Geometry: final body of the model. Coordinates: model frame, mm. A direction names the side the tool comes from. Round coordinates to 2 decimals unless told otherwise and drop trailing zeros. Write each loop counter-clockwise with the first axis right and the second up, starting at its lowest first coordinate (ties: lowest second). Pieces come first, ordered by that corner, then holes. Notation, with made-up numbers: (27, 5) - (33, 5) arc R12 cw to (33, 23) - close; hole circle Ø6 at (79, -22.75). An arc over 180 degrees is marked (long way). Write each question's results on one line, items separated by ' | '.
Autodesk Inventor part; units mm, degrees
ref_plane "Work Plane1" through (0, 10, 0) normal (0, 1, 0) x (-1, 0, 0)
ref_plane "YZ Plane" through (0, 0, 0) normal (1, 0, 0) x (0, 1, 0)
ref_plane "XY Plane" through (0, 0, 0) normal (0, 0, 1) x (1, 0, 0)
sketch "Sketch1" plane through (0, 0, 0) normal (1, 0, 0) x (0, 1, 0)
  circle A0 centre (0, 0) radius 16
  dimension "d0" = 32
extrude "Extrusion1" add sketch "Sketch1" along normal blind 15
sketch "Sketch2" plane through (15, 0, 0) normal (1, 0, 0) x (0, 0, -1)
  circle A0 centre (0, 0) radius 17.5
  dimension "d3" = 35
extrude "Extrusion2" add sketch "Sketch2" along normal blind 5
sketch "Sketch3" plane through (20, 0, 0) normal (1, 0, 0) x (0, 0, -1)
  circle A0 centre (0, 0) radius 10
  dimension "d6" = 20
extrude "Extrusion3" add sketch "Sketch3" along normal blind 10
sketch "Sketch4" plane through (30, 0, 0) normal (1, 0, 0) x (0, 0, -1)
  circle A0 centre (0, 0) radius 4.5
  dimension "d9" = 9
extrude "Extrusion4" cut sketch "Sketch4" against normal blind 58
thread "Thread1"
chamfer "Chamfer1" distance 1 angle 45 1 edges at (0, -16, 0)
ref_plane "Work Plane1" through (0, 10, 0) normal (0, 1, 0) x (-1, 0, 0)
sketch "Sketch5" plane through (0, 10, 0) normal (0, 1, 0) x (-1, 0, 0)
  circle A0 centre (-24.773, 0) radius 2.5
  point P0 (0, 0)
  dimension "d19" = 5
extrude "Extrusion5" cut sketch "Sketch5" against normal blind 27.5
thread "Thread2"
chamfer "Chamfer2" distance 1 angle 45 2 edges at (20, 0, 17.5) (30, 0, 10)
properties part number "sprocet adaptor"
Q1. Section query A-A, the plane z = 0. Give the number of separate pieces and of enclosed holes in the cut face, plus the area to 3 significant figures.
Answer block:
separate pieces: 4 | enclosed holes: 0 | area: 527 mm2
Q2. Pin query (flat end, axial travel): pin 1 (4 mm diameter, centred on x = 12.5, z = 1.5, fed in from +Y); pin 2 (1 mm diameter, centred on x = 23, y = -1.5, fed in from -Z); pin 3 (4 mm diameter, centred on x = 17.5, y = 13, fed in from -Z); pin 4 (17.5 mm diameter, centred on y = 5, z = 7.5, fed in from -X). Return the tip coordinate at first contact, or that it passes through.
Answer block:
pin 1: y = 16 | pin 2: z = -9.95 | pin 3: z = -13.61 | pin 4: x = 0
Q3. Section query D-D, the plane x = 28. Return loops of the section in (y, z), plus the area to 3 significant figures.
Answer block:
outline: circle Ø20 at (0, 0); hole circle Ø9 at (0, 0) | area: 251 mm2
Q4. Section query B-B, the plane y = 0. Return loops of the section in (x, z), plus the area to 3 significant figures.
Answer block:
outline: (0, -15) - (1, -16) - (15, -16) - (15, -17.5) - (19, -17.5) - (20, -16.5) - (20, -10) - (29, -10) - (30, -9) - (30, -4.5) - (0, -4.5) - close; (0, 4.5) - (30, 4.5) - (30, 9) - (29, 10) - (20, 10) - (20, 16.5) - (19, 17.5) - (15, 17.5) - (15, 16) - (1, 16) - (0, 15) - close | area: 582 mm2
Q5. Section query C-C, the plane x = 23. Return loops of the section in (y, z), plus the area to 3 significant figures.
Answer block:
outline: (-9.84, -1.76) arc R10 ccw to (9.84, -1.76) - (4.14, -1.76) arc R4.5 cw to (-4.14, -1.76) - close; (-9.84, 1.76) - (-4.14, 1.76) arc R4.5 cw to (4.14, 1.76) - (9.84, 1.76) arc R10 ccw to start | area: 211 mm2
Q6. Ray query, line 1 along X through (y, z) = (-8, 0); line 2 along Z through (x, y) = (5.5, -4); line 3 along X through (y, z) = (6, 11). Return the intervals inside material, ascending.
Answer block:
line 1: 0 to 22.27, 27.27 to 30 | line 2: -15.49 to -2.06, 2.06 to 15.49 | line 3: 0 to 20
Q7. Mould query, pull axis Z, two halves, no side actions, for faces 4 (the cylindrical face through (7.9, -3.47, 15.62)), 5 (the flat face through (0, 3, 4)), 6 (the cylindrical face through (22.39, -6.83, 0.75)). Classes: pulls with the +Z half, pulls with the -Z half, needs draft (parallel to the pull), parting line crosses it, or undercut.
Answer block:
face 4: parting line crosses it | face 5: needs draft | face 6: undercut
Q8. Access query for faces 1 (the cylindrical face through (24.437, 8.872, -4.614)), 2 (the flat face through (15, -14.2, -7.7)), 3 (the cylindrical face through (23.62, 6.91, -2.22)). Directions: +Z, -Z, +X, -X, +Y, -Y. A direction counts if a zero-diameter tool reaches every point of the face in a straight line with its end or side. Return the directions, or none.
Answer block:
face 1: +X | face 2: -X | face 3: +Y, -Y
